```python
from build123d import *

# Parameters (mm, degrees)
F0_W     = 127
F0_H     = 12.7
F0_W_2   = 635
F0_H_2   = 126.9999911487
F0_R     = 101.6
F0_H_3   = 177.8000088513
F1_DEPTH = 12.7


# Not quite as in the source:
# - a feature names something its author has since deleted; it is built from what else it names


with BuildPart() as f1:
    # F0 (on Top) → F1 (new body)
    with BuildSketch(Plane.XY):
        with BuildLine():
            ThreePointArc((-444.8386187891, 967.019580251), (-588.5227167262, 907.5036781881), (-648.0386187891, 763.819580251))
            Line((-648.0386187891, 763.819580251), (-648.0386187891, -556.980419749))
            Line((-648.0386187891, -556.980419749), (-648.0386187891, -563.330419749))
            Line((-648.0386187891, -563.330419749), (164.7613812109, -563.330419749))
            Line((164.7613812109, -563.330419749), (164.7613812109, -556.980419749))
            Line((164.7613812109, -556.980419749), (164.7613812109, 763.819580251))
            ThreePointArc((164.7613812109, 763.819580251), (105.245479148, 907.5036781881), (-38.4386187891, 967.019580251))
            Line((-38.4386187891, 967.019580251), (-444.8386187891, 967.019580251))
        make_face()
        with Locations((-533.7386187891, -353.780419749)):
            Rectangle(F0_W, F0_H, mode=Mode.SUBTRACT)
        with Locations((50.4613812109, -353.780419749)):
            Rectangle(F0_W, F0_H, mode=Mode.SUBTRACT)
        Polygon((75.8613812109, -48.980419749), (-559.1386187891, -48.980419749), (-559.1386187891, 90.719580251), (-559.1386187891, 141.519580251), (-559.1386187891, 319.319580251), (75.8613812109, 319.319580251), (75.8613812109, 141.519580251), (75.8613812109, 90.719580251), align=None, mode=Mode.SUBTRACT)
        with Locations((-241.6386187891, 433.6195758253)):
            Rectangle(F0_W_2, F0_H_2, mode=Mode.SUBTRACT)
        with Locations((-241.6386187891, 843.8264727592)):
            Circle(F0_R, mode=Mode.SUBTRACT)
        with Locations((-241.6386187891, 636.8195758253)):
            Rectangle(F0_W_2, F0_H_3, mode=Mode.SUBTRACT)
    extrude(amount=F1_DEPTH)


solid = f1.part
```
Could you check a few things on this model? Use its own coordinates, in mm. Coordinates: 2 decimals unless noted, no trailing zeros. Write each loop counter-clockwise with the first axis right and the second up, starting at its lowest first coordinate (ties: lowest second). Pieces come first, ordered by that corner, then holes. Notation, with made-up numbers: (-11, 25.5) -> (36, 25.5) arc R5 cw to (36, 30.5) -> close; hole circle Ø2 at (16, 19.25). An arc over 180 degrees is marked (long way). Return JSON: item names as keys, results as strings.
(1) I need wall thicknesses on L1, parallel to Y at x = -344.5, z = 2.5; L2, parallel to X at y = 107, z = 11.75; L3, parallel to Y at x = 50, z = 10.5. Which ranges of each line are inside material? Lowest first, please.
Numbers:
{"L1": "y = -563.33 to -48.98, 319.32 to 370.12, 497.12 to 547.92, 725.72 to 967.02", "L2": "x = -648.04 to -559.14, 75.86 to 164.76", "L3": "y = -563.33 to -360.13, -347.43 to -48.98, 319.32 to 370.12, 497.12 to 547.92, 725.72 to 946.76"}
(2) We'd pull the mould along X, two halves only. Please class faces 1 (the flat face through (-247, -128, 12.7)), 2 (the cylindrical face through (-316.522, 912.493, 6.261)), 3 (the cylindrical face through (-586.934, 909.075, 6.261)), 4 (the cylindrical face through (106.817, 905.915, 6.261)): +X half, -X half, draft (parallel to the pull), parting line (faces both ways), or undercut.
Numbers:
{"face 1": "draft", "face 2": "undercut", "face 3": "-X half", "face 4": "+X half"}
(3) Imagine slicing it at D-D, the plane z = 7.5. Please give me the cut outline in (x, y).
Numbers:
{"outline": "(-648.04, -563.33) -> (164.76, -563.33) -> (164.76, 763.82) arc R203.2 ccw to (-38.44, 967.02) -> (-444.84, 967.02) arc R203.2 ccw to (-648.04, 763.82) -> close; hole (-597.24, -360.13) -> (-470.24, -360.13) -> (-470.24, -347.43) -> (-597.24, -347.43) -> close; hole (-559.14, -48.98) -> (75.86, -48.98) -> (75.86, 319.32) -> (-559.14, 319.32) -> close; hole (-559.14, 370.12) -> (75.86, 370.12) -> (75.86, 497.12) -> (-559.14, 497.12) -> close; hole (-559.14, 547.92) -> (75.86, 547.92) -> (75.86, 725.72) -> (-559.14, 725.72) -> close; hole circle Ø203.2 at (-241.64, 843.83); hole (-13.04, -360.13) -> (113.96, -360.13) -> (113.96, -347.43) -> (-13.04, -347.43) -> close"}
(4) Imagine slicing it at B-B, the plane x = -370. Please give me the cut outline in (y, z), then the cut area to 3 significant figures.
Numbers:
{"outline": "(-563.33, 0) -> (-48.98, 0) -> (-48.98, 12.7) -> (-563.33, 12.7) -> close; (319.32, 0) -> (370.12, 0) -> (370.12, 12.7) -> (319.32, 12.7) -> close; (497.12, 0) -> (547.92, 0) -> (547.92, 12.7) -> (497.12, 12.7) -> close; (725.72, 0) -> (967.02, 0) -> (967.02, 12.7) -> (725.72, 12.7) -> close", "area": "10,900 mm2"}
(5) Imagine slicing it at C-C, the plane x = -486. Please give me the cut outline in (y, z), then the cut area to 3 significant figures.
Numbers:
{"outline": "(-563.33, 0) -> (-360.13, 0) -> (-360.13, 12.7) -> (-563.33, 12.7) -> close; (-347.43, 0) -> (-48.98, 0) -> (-48.98, 12.7) -> (-347.43, 12.7) -> close; (319.32, 0) -> (370.12, 0) -> (370.12, 12.7) -> (319.32, 12.7) -> close; (497.12, 0) -> (547.92, 0) -> (547.92, 12.7) -> (497.12, 12.7) -> close; (725.72, 0) -> (962.81, 0) -> (962.81, 12.7) -> (725.72, 12.7) -> close", "area": "10,700 mm2"}
(6) Imagine slicing it at A-A, the plane y = 673.5. Please give me the cut outline in (x, z), then the cut area to 3 significant figures.
Numbers:
{"outline": "(-648.04, 0) -> (-559.14, 0) -> (-559.14, 12.7) -> (-648.04, 12.7) -> close; (75.86, 0) -> (164.76, 0) -> (164.76, 12.7) -> (75.86, 12.7) -> close", "area": "2,260 mm2"}
(7) I'm going to push flat-ended pins straight in: pin 1 (3 mm diameter, centred on x = 81, z = 7.5, fed in from +Y); pin 2 (4 mm diameter, centred on x = -505.5, z = 8.5, fed in from +Y); pin 3 (4 mm diameter, centred on x = 75.5, z = 8, fed in from +Y). Where does each tip first touch, or does it pass through?
Numbers:
{"pin 1": "stops at y = 929.29", "pin 2": "stops at y = 958.37", "pin 3": "stops at y = 933.41"}
